For this review, use the dimensioned drawing (mm, ordinates from the lowest corner) and the shaded views. A direction names the side the tool comes from. Coordinates: 2 decimals unless noted, no trailing zeros. Write each loop counter-clockwise with the first axis right and the second up, starting at its lowest first coordinate (ties: lowest second). Pieces come first, ordered by that corner, then holes. Notation, with made-up numbers: (30, 87.25) - (79, 87.25) arc R21 ccw to (79, 121.25) - close; hole circle Ø6 at (30, 12.25). An arc over 180 degrees is marked (long way). Put each result on its own line as item: value.
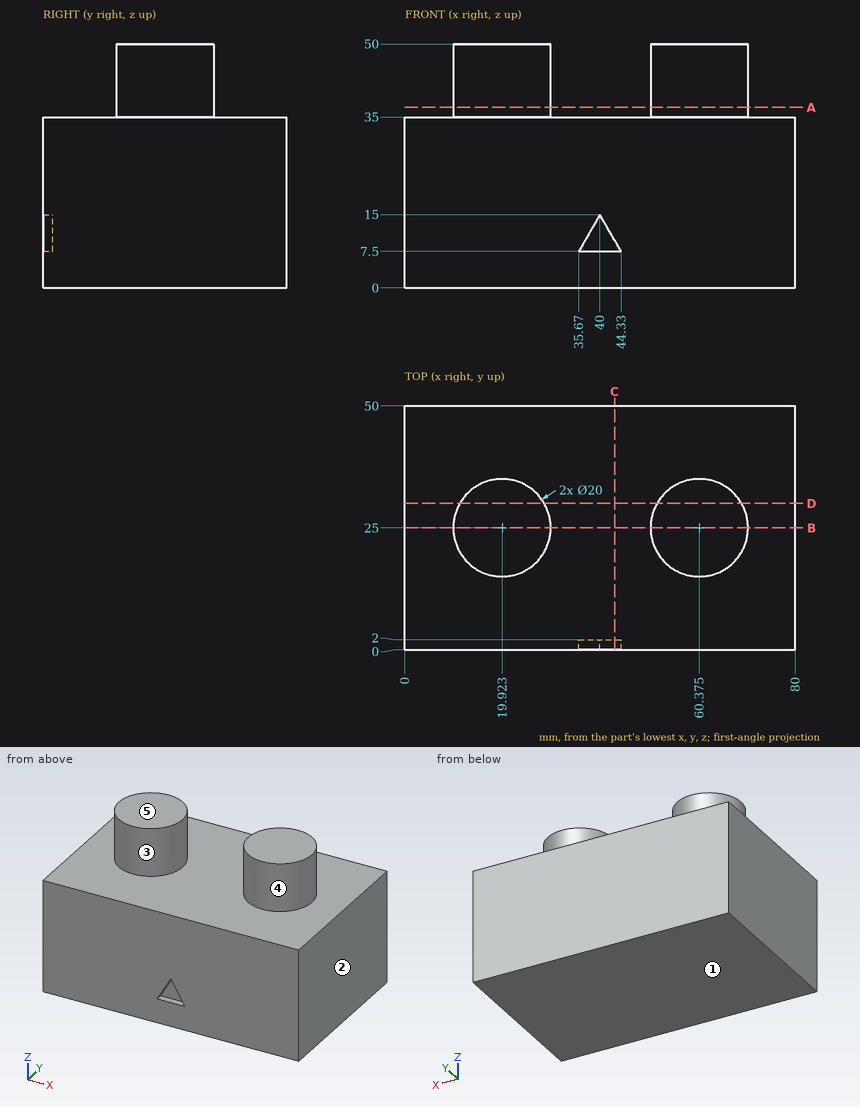
1. Machinability: for the marked faces 4 and 5, which of the approach directions +Z, -Z, +X, -X, +Y, -Y give a long, thin tool a straight path to every point of the face, cutting with its end or side? Answer none if there is none.
Determined:
face 4: +Z
face 5: +Z, +X, -X, +Y, -Y
2. Consider section C-C on x = 43. State the section outline as (y, z) points.
Determined:
outline: (0, 0) - (50, 0) - (50, 35) - (0, 35) - (0, 9.8) - (2, 9.8) - (2, 7.5) - (0, 7.5) - close
3. Consider section B-B on y = 25. State the section outline as (x, z) points (1 decimal).
Determined:
outline: (0, 0) - (80, 0) - (80, 35) - (70.4, 35) - (70.4, 50) - (50.4, 50) - (50.4, 35) - (29.9, 35) - (29.9, 50) - (9.9, 50) - (9.9, 35) - (0, 35) - close
4. For pin 1 Ø1.5 at (x, z) = (22, 40) entering from -Y; pin 2 Ø6 at (x, y) = (31, 34.5) entering from +Z; pin 3 Ø1 at (y, z) = (30, 38.5) entering from +X (1 decimal), all flat-tipped, find the tip position at first contact; note any pin that passes through.
Determined:
pin 1: stops at y = 15.09
pin 2: stops at z = 35
pin 3: stops at x = 69.3
5. Consider section D-D on y = 30. State the section outline as (x, z) points (1 decimal).
Determined:
outline: (0, 0) - (80, 0) - (80, 35) - (69, 35) - (69, 50) - (51.7, 50) - (51.7, 35) - (28.6, 35) - (28.6, 50) - (11.3, 50) - (11.3, 35) - (0, 35) - close
6. The part is to be moulded in two halves that separate along X. For the marked faces 1, 2 and 3, say which applies: +X half, -X half, draft (parallel to the pull), parting line (faces both ways), or undercut.
Determined:
face 1: draft
face 2: +X half
face 3: undercut
7. To check wall thickness, follow probe 1 along Z at (x, y) = (11, 20); probe 2 along X at (y, z) = (30.5, 42) (1 decimal); probe 3 along X at (y, z) = (32.5, 47.5) (1 decimal). State the ranges of each line that lie inside material, in increasing order.
Determined:
probe 1: z = 0 to 35
probe 2: x = 11.6 to 28.3, 52 to 68.7
probe 3: x = 13.3 to 26.5, 53.8 to 67
8. Consider section A-A on z = 37. State the section outline as (x, y) points (1 decimal).
Determined:
outline: circle Ø20 at (19.9, 25); circle Ø20 at (60.4, 25)
